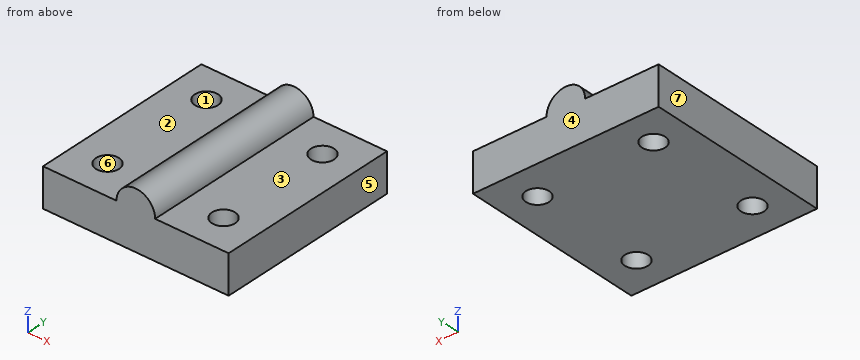
from build123d import *

# Parameters (mm, degrees)
F0_W     = 48
F0_H     = 48
F1_DEPTH = 10
F3_DEPTH = 48
F5_D     = 6


with BuildPart() as f1:
    # F0 (on Top) → F1 (new body)
    with BuildSketch(Plane.XY):
        with Locations((24, 24)):
            Rectangle(F0_W, F0_H)
    extrude(amount=F1_DEPTH)

    # F2 (on face) → F3 (join, through all)
    with BuildSketch(Plane.XZ):
        with BuildLine():
            Line((19, 10), (29, 10))
            ThreePointArc((29, 10), (24, 15), (19, 10))
        make_face()
    extrude(amount=-F3_DEPTH)

    # F5 (through all)
    with Locations(Plane(origin=(0, 0, 0), x_dir=(1, 0, 0), z_dir=(0, 0, -1))):
        with Locations((9, -9), (9, -39), (39, -39), (39, -9)):
            Hole(F5_D / 2)


solid = f1.part
Part model, mm, in its own coordinate system. Face numbers are marked on the shaded views. A direction names the side the tool comes from. Give positions to 0.01 mm unless a question says otherwise; leave off trailing zeros. Order: outer loops, then holes, each group sorted by start corner. A loop starts at its lowest first (then second) coordinate and runs counter-clockwise, first axis right, second up. Notation, with made-up numbers: (20, 2.25) - (59, 2.25) arc R13 cw to (59, 20.25) - close; hole circle Ø4 at (36.25, 12.25). An arc over 180 degrees is marked (long way). Use a Markdown table: item, result.
1) 3-axis set-ups, long thin cutter, end or side, ignore diameter. For the marked faces 1, 2 and 3: which of +Z, -Z, +X, -X, +Y, -Y reach the whole face in a straight line?
Checked values:
| item | result |
|---|---|
| face 1 | +Z, -Z |
| face 2 | +Z, -X, +Y, -Y |
| face 3 | +Z, +X, +Y, -Y |
2) Saw through at A-A on x = 9. List the corners of the cut face in (y, z).
Checked values:
| item | result |
|---|---|
| outline | (0, 0) - (6, 0) - (6, 10) - (0, 10) - close; (12, 0) - (36, 0) - (36, 10) - (12, 10) - close; (42, 0) - (48, 0) - (48, 10) - (42, 10) - close |
3) Probe L1, parallel to Y at x = 9, z = 7.75; L2, parallel to Z at x = 3.5, y = 18. List the from-to ranges inside material, lowest first. Write a range as from..to.
Checked values:
| item | result |
|---|---|
| L1 | 0..6, 12..36, 42..48 |
| L2 | 0..10 |
4) Saw through at B-B on y = 9. List the corners of the cut face in (x, z), plus the area to 3 significant figures.
Checked values:
| item | result |
|---|---|
| outline | (0, 0) - (6, 0) - (6, 10) - (0, 10) - close; (12, 0) - (36, 0) - (36, 10) - (29, 10) arc R5 ccw to (19, 10) - (12, 10) - close; (42, 0) - (48, 0) - (48, 10) - (42, 10) - close |
| area | 399 mm² |
5) Flat gauge pins, fed straight in: P1, Ø10, axis at x = 15.5, y = 39.5, coming from the +Z side; P2, Ø1.5, axis at y = 32, z = 11.5, coming from the +X side; P3, Ø5.5, axis at x = 37.5, y = 21.5, coming from the +Z side. Where does each tip first touch, or does it go through?
Checked values:
| item | result |
|---|---|
| P1 | z = 13.57 |
| P2 | x = 28.94 |
| P3 | z = 10 |
6) Saw through at D-D on y = 30. List the corners of the cut face in (x, z).
Checked values:
| item | result |
|---|---|
| outline | (0, 0) - (48, 0) - (48, 10) - (29, 10) arc R5 ccw to (19, 10) - (0, 10) - close |
7) Saw through at C-C on z = 3. List the corners of the cut face in (x, y).
Checked values:
| item | result |
|---|---|
| outline | (0, 0) - (48, 0) - (48, 48) - (0, 48) - close; hole circle Ø6 at (9, 9); hole circle Ø6 at (9, 39); hole circle Ø6 at (39, 9); hole circle Ø6 at (39, 39) |
8) Two-plate mould, pull along X, no slides. Class the marked faces 4, 5, 6 and 7: +X half, -X half, draft (parallel to the pull), parting line (faces both ways), or undercut.
Checked values:
| item | result |
|---|---|
| face 4 | draft |
| face 5 | +X half |
| face 6 | undercut |
| face 7 | -X half |
